```python
from build123d import *

# Parameters (mm, degrees)
SKETCH4_W               = 104
SKETCH4_H               = 104
BOSS_EXTRUDE2_DEPTH     = 57.5
BOSS_EXTRUDE2_TAPER     = 23
SKETCH6_R               = 25
CUT_EXTRUDE1_DEPTH      = 179.5
CUT_EXTRUDE_THIN1_START = 10
CUT_EXTRUDE_THIN1_DEPTH = 10
CUT_EXTRUDE3_DEPTH      = 124
SKETCH10_R              = 35
CUT_EXTRUDE4_DEPTH      = 10
FILLET9_R               = 15
FILLET10_R              = 15
BOSS_EXTRUDE5_DEPTH     = 10
FILLET16_R              = 5
FILLET17_R              = 5
CUT_EXTRUDE6_DEPTH      = 10
CUT_EXTRUDE7_DEPTH      = 10


with BuildPart() as part:
    # Sketch4 → Boss-Extrude2 (new body)
    with BuildSketch(Plane.XY):
        with Locations((52, 52)):
            Rectangle(SKETCH4_W, SKETCH4_H)
    boss_extrude2 = extrude(amount=BOSS_EXTRUDE2_DEPTH, taper=BOSS_EXTRUDE2_TAPER)

    # Mirror2: Boss-Extrude2 across plane
    add(boss_extrude2.mirror(Plane(origin=(0, 0, 57.5), x_dir=(1, 0, 0), z_dir=(0, 0, -1))))

    # Sketch6 → Cut-Extrude1 (cut)
    with BuildSketch(Plane.XY.offset(115)):
        with Locations((52, 52)):
            Circle(SKETCH6_R)
    extrude(amount=-CUT_EXTRUDE1_DEPTH, mode=Mode.SUBTRACT)

    # Sketch8 → Cut-Extrude-Thin1 (cut)
    with BuildSketch(Plane.XY.offset(CUT_EXTRUDE_THIN1_START)):
        with BuildLine():
            ThreePointArc((52, 17), (76.748737342, 76.748737342), (17, 52))
            Line((17, 52), (7, 52))
            ThreePointArc((7, 52), (83.819805153, 83.819805153), (52, 7))
            Line((52, 7), (52, 17))
        make_face()
        with BuildLine():
            ThreePointArc((52, 27), (69.67766953, 69.67766953), (27, 52))
            Line((27, 52), (17, 52))
            ThreePointArc((17, 52), (76.748737342, 76.748737342), (52, 17))
            Line((52, 17), (52, 27))
        make_face()
    extrude(amount=-CUT_EXTRUDE_THIN1_DEPTH, mode=Mode.SUBTRACT)

    # Sketch9 → Cut-Extrude3 (cut)
    with BuildSketch(Plane(origin=(0, 0, 0), x_dir=(-1, 0, 0), z_dir=(0, 0, -1))):
        Polygon((-27, 52), (0, 52), (0, 0), (-52, 0), (-52, 27), (-52, 52), align=None)
    extrude(amount=-CUT_EXTRUDE3_DEPTH, mode=Mode.SUBTRACT)

    # Sketch10 → Cut-Extrude4 (cut)
    with BuildSketch(Plane.XY.offset(115)):
        with Locations((52, 52)):
            Circle(SKETCH10_R)
    extrude(amount=-CUT_EXTRUDE4_DEPTH, mode=Mode.SUBTRACT)

    # Fillet9
    fillet9_edges = [part.edges().sort_by_distance(p)[0] for p in [
        (65.796349034, 24.407301932, 57.5),
    ]]
    fillet(fillet9_edges, radius=FILLET9_R)

    # Fillet10
    fillet10_edges = [part.edges().sort_by_distance(p)[0] for p in [
        (24.407301932, 65.796349034, 57.5),
        (52, 79.592698068, 57.5),
        (79.592698068, 51.352297169, 57.5),
    ]]
    fillet(fillet10_edges, radius=FILLET10_R)

    # Sketch12 → Boss-Extrude5 (add)
    with BuildSketch(Plane(origin=(0, 0, 0), x_dir=(-1, 0, 0), z_dir=(0, 0, -1))):
        Polygon((-104, 104), (0, 104), (0, 52), (-3, 52), (-3, 101), (-101, 101), (-101, 3), (-52, 3), (-52, 0), (-104, 0), align=None)
    extrude(amount=BOSS_EXTRUDE5_DEPTH)

    # Fillet16
    fillet16_edges = [part.edges().sort_by_distance(p)[0] for p in [
        (78, 0, 0),
    ]]
    fillet(fillet16_edges, radius=FILLET16_R)

    # Fillet17
    fillet17_edges = [part.edges().sort_by_distance(p)[0] for p in [
        (0, 78, 0),
        (52, 104, 0),
        (104, 52.052287852, 0),
    ]]
    fillet(fillet17_edges, radius=FILLET17_R)

    # Sketch14 → Cut-Extrude6 (cut)
    with BuildSketch(Plane(origin=(0, 0, 0), x_dir=(-1, 0, 0), z_dir=(0, 0, -1))):
        with BuildLine():
            Line((-94.485281374, 98.727922061), (-83.878679656, 88.121320344))
            ThreePointArc((-83.878679656, 88.121320344), (-83.878679656, 83.878679656), (-88.121320344, 83.878679656))
            Line((-88.121320344, 83.878679656), (-98.727922061, 94.485281374))
            ThreePointArc((-98.727922061, 94.485281374), (-98.727922061, 98.727922061), (-94.485281374, 98.727922061))
        make_face()
    extrude(amount=-CUT_EXTRUDE6_DEPTH, mode=Mode.SUBTRACT)

    # Sketch15 → Cut-Extrude7 (cut)
    with BuildSketch(Plane(origin=(0, 0, 0), x_dir=(-1, 0, 0), z_dir=(0, 0, -1))):
        with BuildLine():
            Line((-20.170334378, 88.072306309), (-9.56373266, 98.678908027))
            ThreePointArc((-9.56373266, 98.678908027), (-5.321091973, 98.678908027), (-5.321091973, 94.43626734))
            Line((-5.321091973, 94.43626734), (-15.927693691, 83.829665622))
            ThreePointArc((-15.927693691, 83.829665622), (-20.170334378, 83.829665622), (-20.170334378, 88.072306309))
        make_face()
        with BuildLine():
            Line((-83.832077939, 15.925281374), (-94.438679656, 5.318679656))
            ThreePointArc((-94.438679656, 5.318679656), (-98.681320344, 5.318679656), (-98.681320344, 9.561320344))
            Line((-98.681320344, 9.561320344), (-88.074718626, 20.167922061))
            ThreePointArc((-88.074718626, 20.167922061), (-83.832077939, 20.167922061), (-83.832077939, 15.925281374))
        make_face()
    extrude(amount=-CUT_EXTRUDE7_DEPTH, mode=Mode.SUBTRACT)


solid = part.part
```
The model under review builds one solid part; all positions refer to its coordinate system, in mm. A direction names the side the tool comes from. Round coordinates to 2 decimals unless told otherwise and drop trailing zeros. Order: outer loops, then holes, each group sorted by start corner. A loop starts at its lowest first (then second) coordinate and runs counter-clockwise, first axis right, second up. Notation, with made-up numbers: (58.5, 48.25) -> (114.5, 48.25) arc R7 cw to (114.5, 56.25) -> close; hole circle Ø5 at (34.25, -7). An arc over 180 degrees is marked (long way). One line per item, written item: value. Start each with the question number.
Q1. Take a section at D-D (y = 73.5). Write out the cut boundary in (x, z).
Q2. Machinability: for faces 5 (the face through (93.194, 52.728, 89.542)), 6 (the face through (23.11, 66.83, 57.42)), 7 (the face through (74, 92, 0)), 8 (the face through (72.429, 11.008, 25.933)), 9 (the face through (51.272, 93.194, 89.542)), which of the approach directions +Z, -Z, +X, -X, +Y, -Y give a long, thin tool a straight path to every point of the face, cutting with its end or side? Answer none if there is none.
Q3. Clearance check with flat-ended pins moving along their axes: pin 1 Ø5 at (x, y) = (88, 13) entering from -Z; pin 2 Ø8 at (y, z) = (19, 22.5) entering from -X; pin 3 Ø2 at (y, z) = (27, 26.5) entering from +X. State where each tip first meets the part, or that it passes through.
Q4. Wall thickness on line 1 (Z direction, x = 76, y = 90.5); line 2 (Y direction, x = 65.5, z = 106.5); line 3 (Z direction, x = 64, y = 29.5): over which ranges is each line inside the solid? List them lowest first.
Q5. Mouldability with a two-part tool opening along Y and no side actions: class faces 1 (the face through (70, 70, 105)), 2 (the face through (72.586, 10.806, 89.542)), 3 (the face through (10.806, 71.858, 89.542)), 4 (the face through (77, 3, -5)) as released by +Y, released by -Y, zero draft, split by the parting line, or undercut.
Q6. Take a section at A-A (x = 12.5). Write out the cut boundary in (y, z), and give its area (3 significant figures).
Q7. Take a section at B-B (y = 35.5). Write out the cut boundary in (x, z).
Q8. Take a section at C-C (z = 43). Write out the cut boundary in (x, y).
Reported:
1. outline: (0, -10) -> (3, -10) -> (3, 0) -> (12.47, 0) -> (12.47, 10) -> (39.24, 10) -> (39.24, 105) -> (24.38, 105) -> (24.38, 115) -> (0, 115) -> (21.92, 63.36) arc R15 cw to (21.92, 51.64) -> (0.4, 0.94) arc R5 ccw to (0, -1.02) -> close; (64.76, 10) -> (91.53, 10) -> (91.53, 0) -> (101, 0) -> (101, -10) -> (104, -10) -> (104, -1.02) arc R5 ccw to (103.6, 0.94) -> (82.08, 51.64) arc R15 cw to (82.08, 63.36) -> (104, 115) -> (79.62, 115) -> (79.62, 105) -> (64.76, 105) -> close
2. face 5: +X, +Y, -Y
2. face 6: -X, +Y, -Y
2. face 7: -Z
2. face 8: +X, -X, -Y
2. face 9: +X, -X, +Y
3. pin 1: stops at z = 0
3. pin 2: stops at x = 52
3. pin 3: stops at x = 93.18
4. line 1: z = 0 to 31.8, 83.2 to 115
4. line 2: y = 3.61 to 19.71, 84.29 to 100.39
4. line 3: z = 10 to 105
5. face 1: undercut
5. face 2: released by -Y
5. face 3: zero draft
5. face 4: undercut
6. outline: (52, 10) -> (73.56, 10) -> (73.56, 0) -> (87.26, 0) -> (87.26, 10) -> (95.74, 10) -> (95.74, 0) -> (101, 0) -> (101, -10) -> (104, -10) -> (104, -1.02) arc R5 ccw to (103.6, 0.94) -> (91.5, 29.45) -> (52, 29.45) -> close; (52, 85.55) -> (91.5, 85.55) -> (104, 115) -> (52, 115) -> close
6. area: 2,420 mm2
7. outline: (70.78, 10) -> (93.87, 10) -> (93.87, 0) -> (101, 0) -> (101, -10) -> (104, -10) -> (104, -1.02) arc R5 ccw to (103.6, 0.94) -> (82.08, 51.64) arc R15 cw to (82.08, 63.36) -> (104, 115) -> (82.87, 115) -> (82.87, 105) -> (70.78, 105) -> close
8. outline: (18.25, 52) -> (27, 52) arc R25 cw (long way) to (52, 27) -> (52, 18.25) -> (85.75, 18.25) -> (85.75, 85.75) -> (18.25, 85.75) -> close
